Could you check a few things on this model? Use its own coordinates, in mm. A direction names the side the tool comes from. Give positions to 0.01 mm unless a question says otherwise; leave off trailing zeros. Loops run counter-clockwise (first coordinate to the right, second up) from the corner with the lowest first, then second, coordinate; pieces in that order, holes last. Notation, with made-up numbers: M 15.5,86.25 L 28.5,86.25 A13 ccw 28.5,109.25 Z; hole C 22,4.25 d2. An arc over 180 degrees is marked long. Answer in a Markdown table with one row per item. Add a question column.
1. Which directions (+Z, -Z, +X, -X, +Y, -Y) give clear straight access to the entire face, cutting with the end or side of a thin tool? Please do faces 4 (the flat face through (15, 20, -14)), 5 (the cylindrical face through (37.608, 17.847, -2.343)), 6 (the flat face through (10.73, -16.01, -31.01)).
2. I'm going to push flat-ended pins straight in: pin 1 Ø6 at (x, z) = (-8.5, 20.5) entering from +Y; pin 2 Ø13 at (x, y) = (53, -30.5) entering from -Z; pin 3 Ø4 at (y, z) = (-30, -8) entering from -X; pin 4 Ø7 at (y, z) = (0, 34) entering from +X. Where does each tip first touch, or does it pass through?
3. Thinking about a two-plate mould opening in Z: for faces 1 (the cylindrical face through (22, -39.01, 43.54)), 2 (the flat face through (29, -38, -38)), 3 (the cylindrical face through (12.46, -28.02, -10.72)), which applies, released by +Z, released by -Z, zero draft, split by the parting line, or undercut?
4. If we section it at D-D on y = 0: Count the separate pieces of the cut face and the enclosed holes in it, then the cut area to 3 significant figures.
5. If we section it at B-B on z = 34: List the corners of the cut face in (x, y) for me.
6. I need wall thicknesses on line 1 along Z through (x, y) = (24.5, -46); line 2 along Z through (x, y) = (14, 0.5); line 3 along Y through (x, z) = (22, -10.5). Which ranges of each line are inside material? Lowest first, please. Write a range as from..to.
7. If we section it at A-A on x = 25: List the corners of the cut face in (y, z) for me, then the cut area to 3 significant figures.
8. If we section it at C-C on y = 13: List the corners of the cut face in (x, z) for me.
```python
from build123d import *
from OCP.BRepFilletAPI import BRepFilletAPI_MakeFillet

# Parameters (mm, degrees)
EXTRUDE_1_DEPTH      = 15
EXTRUDE_START        = 2
SKETCH_2_R           = 24
EXTRUDE_2_DEPTH      = 75
EXTRUDE_START_2      = -75
SKETCH_3_R           = 17.5
EXTRUDE_3_DEPTH      = 90
SKETCH_4_W           = 53
SKETCH_4_H           = 96
EXTRUDE_4_DEPTH      = 10
FILLET_1_R1          = 2
FILLET_1_R2          = 10
SKETCH_5_R           = 10
EXTRUDE_5_DEPTH      = 2
SKETCH_6_R           = 5.5
CUT_EXTRUDE_1_DEPTH  = 122.128031438
EXTRUDE_6_DEPTH      = 10
RIB_1_REACH          = 114.018
SKETCH_8_WALL_W      = 244.903673704
SKETCH_8_WALL_H      = 10
SKETCH_12_R          = 21
CUT_EXTRUDE_3_DEPTH  = 12
SKETCH_13_R          = 18
CUT_EXTRUDE_4_DEPTH  = 56
HOLE_WIZARD_G1_2_1_D = 19
HOLE_WIZARD_M10_1_D  = 8.5
RIB_START            = -5
RIB_13_DEPTH         = 10


with BuildPart() as part:
    # Sketch 1 → Extrude 1 (new body)
    with BuildSketch(Plane(origin=(0, 0, 0), x_dir=(0, 0, -1), z_dir=(1, 0, 0))):
        with BuildLine():
            Line((15.882352941, 25.45095018), (40.352941176, 10.180380072))
            ThreePointArc((40.352941176, 10.180380072), (46, 0), (40.352941176, -10.180380072))
            Line((40.352941176, -10.180380072), (15.882352941, -25.45095018))
            ThreePointArc((15.882352941, -25.45095018), (0, -30), (-15.882352941, -25.45095018))
            Line((-15.882352941, -25.45095018), (-40.352941176, -10.180380072))
            ThreePointArc((-40.352941176, -10.180380072), (-46, 0), (-40.352941176, 10.180380072))
            Line((-40.352941176, 10.180380072), (-15.882352941, 25.45095018))
            ThreePointArc((-15.882352941, 25.45095018), (0, 30), (15.882352941, 25.45095018))
        make_face()
    extrude(amount=EXTRUDE_1_DEPTH)

    # Sketch 2 → Extrude 2 (add)
    with BuildSketch(Plane.ZY.offset(EXTRUDE_START)):
        Circle(SKETCH_2_R)
    extrude(amount=-EXTRUDE_2_DEPTH)

    # Sketch 3 → Extrude 3 (add)
    with BuildSketch(Plane(origin=(73, 0, 0), x_dir=(0, 0, -1), z_dir=(1, 0, 0)).offset(EXTRUDE_START_2)):
        with Locations(Location((0, 0, 0), (0, 0, 180))):
            Circle(SKETCH_3_R)
    extrude(amount=EXTRUDE_3_DEPTH)



with BuildPart() as body_2:
    # Sketch 4 → Extrude 4 (new body)
    with BuildSketch(Plane(origin=(0, -50, 0), x_dir=(1, 0, 0), z_dir=(0, 1, 0))):
        with Locations((14.5, 0)):
            Rectangle(SKETCH_4_W, SKETCH_4_H)
    extrude(amount=EXTRUDE_4_DEPTH)

    # Fillet 1: one fillet with a radius per group of edges: ONE call of the kernel's fillet builder (fillet() takes one radius for all edges)
    fillet_1_edges_1 = [body_2.edges().sort_by_distance(p)[0] for p in [
        (-12, -45, 48),
        (-12, -45, -48),
    ]]
    fillet_1_edges_2 = [body_2.edges().sort_by_distance(p)[0] for p in [
        (41, -45, -48),
        (41, -45, 48),
    ]]
    fillet_1 = BRepFilletAPI_MakeFillet(body_2.part.solid().wrapped)
    for e in fillet_1_edges_1:
        fillet_1.Add(FILLET_1_R1, e.wrapped)
    for e in fillet_1_edges_2:
        fillet_1.Add(FILLET_1_R2, e.wrapped)
    add(Compound.cast(fillet_1.Shape()), mode=Mode.REPLACE)

    # Sketch 5 → Extrude 5 (add)
    with BuildSketch(Plane(origin=(0, -40, 0), x_dir=(1, 0, 0), z_dir=(0, 1, 0))):
        with Locations(Location((25, 34, 0), (0, 0, 90))):
            Circle(SKETCH_5_R)
    extrude_5 = extrude(amount=EXTRUDE_5_DEPTH)

    # Sketch 6 → Cut-Extrude 1 (cut, through all)
    with BuildSketch(Plane(origin=(0, -38, 0), x_dir=(1, 0, 0), z_dir=(0, 1, 0))):
        with Locations(Location((25, 34, 0), (0, 0, 270))):
            Circle(SKETCH_6_R)
    cut_extrude_1 = extrude(amount=-CUT_EXTRUDE_1_DEPTH, mode=Mode.SUBTRACT)

    # Mirror 1: Extrude 5, Cut-Extrude 1 across plane
    add(extrude_5.mirror(Plane.XY))
    add(cut_extrude_1.mirror(Plane.XY), mode=Mode.SUBTRACT)


with BuildPart() as part_1:
    add(part.part)

    add(body_2.part)  # Extrude 6 merges body 2
    # Sketch 7 → Extrude 6 (add)
    with BuildSketch(Plane.ZY):
        with BuildLine():
            Line((48, -40), (31.147709092, -23.147709092))
            ThreePointArc((31.147709092, -23.147709092), (29.715553271, -19.044672956), (32.036184174, -15.370350156))
            Line((32.036184174, -15.370350156), (15.882352941, -25.45095018))
            ThreePointArc((15.882352941, -25.45095018), (0, -30), (-15.882352941, -25.45095018))
            Line((-15.882352941, -25.45095018), (-32.036184174, -15.370350156))
            ThreePointArc((-32.036184174, -15.370350156), (-29.715553271, -19.044672956), (-31.147709092, -23.147709092))
            Line((-31.147709092, -23.147709092), (-48, -40))
            Line((-48, -40), (-46, -40))
            Line((-46, -40), (46, -40))
            Line((46, -40), (48, -40))
        make_face()
    extrude(amount=-EXTRUDE_6_DEPTH)

    # Sketch 8 wall → Rib 1 (add, up to next)
    with BuildSketch(Plane(origin=(-7, -32, 0), x_dir=(0.529998940003, 0.847998304005, 0), z_dir=(-0.847998304005, 0.529998940003, 0)), mode=Mode.PRIVATE) as rib_1_sk1:
        Rectangle(SKETCH_8_WALL_W, SKETCH_8_WALL_H)
    rib_1_tool1 = extrude(rib_1_sk1.sketch, amount=-RIB_1_REACH, mode=Mode.PRIVATE) - part_1.part
    add(rib_1_tool1.solids().sort_by_distance((-7, -32, 0))[0])

    # Sketch 12 → Cut-Extrude 3 (cut)
    with BuildSketch(Plane.ZY.offset(2)):
        Circle(SKETCH_12_R)
    extrude(amount=-CUT_EXTRUDE_3_DEPTH, mode=Mode.SUBTRACT)

    # Sketch 13 → Cut-Extrude 4 (cut)
    with BuildSketch(Plane.ZY.offset(-10)):
        Circle(SKETCH_13_R)
    extrude(amount=-CUT_EXTRUDE_4_DEPTH, mode=Mode.SUBTRACT)

    # Hole Wizard G1_2 _1 (through all)
    with Locations(Plane.ZY.offset(-66)):
        with Locations((0, 0)):
            Hole(HOLE_WIZARD_G1_2_1_D / 2)

    # Hole Wizard M10 _1 (through all)
    with Locations(Plane.ZY):
        with Locations((34, 0), (-34, 0)):
            Hole(HOLE_WIZARD_M10_1_D / 2)

    # Rib 13: read off the stored shape, not the designer's step
    # Rib 13 outline → Rib 13 (add)
    with BuildSketch(Plane.XY.offset(RIB_START)):
        Polygon((41, -40), (73, -24.001), (73, -23.473389189), (15, -23.473389189), (15, -29.580398915), (10, -29.580398915), (10, -40), align=None)
    extrude(amount=RIB_13_DEPTH)


solid = part_1.part
```
Results:
| question | item | result |
|---|---|---|
| 1 | face 4 | +X |
| 1 | face 5 | -X |
| 1 | face 6 | -Z, +X |
| 2 | pin 1 | y = -40 |
| 2 | pin 2 | z = -5 |
| 2 | pin 3 | x = 0 |
| 2 | pin 4 | through |
| 3 | face 1 | undercut |
| 3 | face 2 | zero draft |
| 3 | face 3 | released by -Z |
| 4 | separate pieces | 4 |
| 4 | enclosed holes | 0 |
| 4 | area | 1,590 mm2 |
| 5 | outline | M -12,-50 L 19.5,-50 L 19.5,-38 L 15,-38 L 15,-40 L 10,-40 L 10,-26 L 0,-26 L 0,-40 L -12,-40 Z; M 0,-14.14 L 15,-14.14 L 15,-4.25 L 0,-4.25 Z; M 0,4.25 L 15,4.25 L 15,14.14 L 0,14.14 Z; M 30.5,-50 L 41,-50 L 41,-40 L 35,-40 L 35,-38 L 30.5,-38 Z |
| 6 | line 1 | -48..-39.48, -28.52..28.52, 39.48..48 |
| 6 | line 2 | -45.99..-38.22, -29.78..-17.99, 17.99..29.78, 38.22..45.99 |
| 6 | line 3 | -50..-40, -21.58..-14.62, 14.62..21.58 |
| 7 | outline | M -50,-48 L -40,-48 L -40,-44 L -38,-44 L -38,-39.5 L -50,-39.5 Z; M -50,-28.5 L -38,-28.5 L -38,-24 L -40,-24 L -40,-5 L -23.47,-5 A24 ccw long -23.47,5 L -40,5 L -40,24 L -38,24 L -38,28.5 L -50,28.5 Z; M -50,39.5 L -38,39.5 L -38,44 L -40,44 L -40,48 L -50,48 Z; hole C 0,0 d36 |
| 7 | area | 1,730 mm2 |
| 8 | outline | M -2,-20.17 L 0,-20.17 L 0,-35.83 L 15,-35.83 L 15,-20.17 L 73,-20.17 L 73,-11.72 L 88,-11.72 L 88,11.72 L 73,11.72 L 73,20.17 L 15,20.17 L 15,35.83 L 0,35.83 L 0,20.17 L -2,20.17 L -2,16.49 L 10,16.49 L 10,12.45 L 66,12.45 L 66,-12.45 L 10,-12.45 L 10,-16.49 L -2,-16.49 Z |
